Verification items for the finished model (mm, model axes). A direction names the side the tool comes from. Coordinates: 2 decimals unless noted, no trailing zeros. Use CSV: the item, a comma, the result in double quotes. Start each with the question number.
1) Tool access check on faces 1 (the flat face through (-256, -6.969, -14)), 2 (the flat face through (17, 4.65, -13)), 3 (the flat face through (-122.2, 29, -14)), 4 (the flat face through (9, -0.35, -13)), 5 (the flat face through (-256.9, -4.719, -11.7)). Record the directions out of +Z, -Z, +X, -X, +Y, -Y that give a thin tool (end or side, any length) a straight path to the whole face; none if there is none.
2) Go/stop test with flat-tipped pins: pin 1 (4.5 mm diameter, centred on y = 12.5, z = -11, fed in from +X); pin 2 (8 mm diameter, centred on x = -131.5, z = -16.5, fed in from +Y); pin 3 (3.5 mm diameter, centred on x = 13.66, z = -13.5, fed in from -Y). Record where each tip stops, or that it passes through.
3) Scan lines: line 1 along X through (y, z) = (29.5, -16); line 2 along Y through (x, z) = (-69.2, -17.5); line 3 along Y through (x, z) = (-67, -7.5). Record each from-to range of solid material in increasing order.
4) Release check for a two-part mould opening along X. For faces 6 (the flat face through (-259.656, -7, -13)), 7 (the flat face through (18.69, 2, -13)), 8 (the flat face through (-200.81, 14, -14)) record: released by +X, released by -X, zero draft, split by the parting line, or undercut.
from build123d import *

# Parameters (mm, degrees)
BOSS_EXTRUDE14_DEPTH            = 15
SKETCH9_W                       = 10.305582395
SKETCH9_H                       = 5
BOSS_EXTRUDE15_DEPTH            = 15
BOSS_EXTRUDE16_START            = -15
BOSS_EXTRUDE16_OUTLINE_R        = 4
BOSS_EXTRUDE16_DEPTH            = 15
FILLET1_R                       = 4
CUT_EXTRUDE2_DEPTH              = 2.25
CUT_EXTRUDE3_DEPTH              = 2.25
F_3_0MM_DOWEL_HOLE1_D           = 3
F_3_0MM_DOWEL_HOLE1_CSINK_D     = 3.05
F_3_0MM_DOWEL_HOLE1_CSINK_ANGLE = 90
SKETCH16_R                      = 1.5
CUT_EXTRUDE4_DEPTH              = 265.853431953


# Read off the part's stored shape, not the designer's step: Boss-Extrude14, Boss-Extrude16
with BuildPart() as part:
    # Boss-Extrude14 outline → Boss-Extrude14 (new body)
    with BuildSketch(Plane(origin=(0, 0, -6), x_dir=(-1, 0, 0), z_dir=(0, 0, -1))):
        with BuildLine():
            Line((249.35, -9.718799499), (249.35, 0.281200501))
            Line((249.35, 0.281200501), (236.35, 2.868680647))
            add(Edge.make_bspline(
                [(113.156309789, 25.751987472), (114.460208978, 25.59959164), (120.100287856, 24.908577179), (128.609098159, 23.664110071), (140.134091586, 21.688830409), (153.008895552, 19.221496185), (168.538046321, 16.015172699), (182.477939999, 13.172125281), (193.559005245, 11.111240975), (201.981640704, 9.637661129), (210.486612866, 8.154956205), (219.063637957, 6.591746422), (227.68151116, 4.874943897), (233.474971, 3.568357951), (236.35, 2.868680647)],
                knots=[0.109458463, 0.109458463, 0.109458463, 0.109458463, 0.130371933, 0.200030506, 0.247022058, 0.318338141, 0.412321245, 0.506304349, 0.553295901, 0.600287453, 0.647279005, 0.694270557, 0.741262109, 0.788253661, 0.788253661, 0.788253661, 0.788253661], degree=3))
            add(Edge.make_bspline(
                [(76.45, 28.125418087), (94.882372903, 27.862574162), (113.156309789, 25.751987472)],
                knots=[0, 0, 0, 0.632722323, 0.632722323, 0.632722323], degree=2))
            add(Edge.make_bspline(
                [(66.284340587, 28.219952736), (67.129544996, 28.219602739), (68.818588071, 28.215923169), (71.36030606, 28.198672488), (73.903160315, 28.169538769), (75.601337427, 28.141603711), (76.45, 28.125418087)],
                knots=[0.875312122, 0.875312122, 0.875312122, 0.875312122, 0.888961276, 0.902610431, 0.916259586, 0.92990874, 0.92990874, 0.92990874, 0.92990874], degree=3))
            add(Edge.make_bspline(
                [(-4.147448422, 10.754973325), (-3.746592061, 11.135583203), (-2.910664688, 11.873123525), (-1.8664669, 12.676265805), (-1.020623492, 13.271741618), (-0.136993775, 13.859475937), (1.465019188, 14.831768722), (3.815921844, 16.045559455), (7.753628889, 17.758192835), (13.256195767, 19.698691993), (21.152959065, 21.952811545), (30.479838242, 24.122904012), (39.4239247, 25.749420494), (47.205771024, 26.831006606), (53.324700432, 27.499051298), (58.631201034, 27.906826379), (62.977570557, 28.125868706), (65.18464413, 28.194929818), (66.284340587, 28.219952736)],
                knots=[0.135157363, 0.135157363, 0.135157363, 0.135157363, 0.162214964, 0.189272566, 0.201061372, 0.214590172, 0.243387768, 0.297502971, 0.351618174, 0.459848579, 0.568078984, 0.676309389, 0.784539795, 0.838654997, 0.8927702, 0.946885402, 0.973943004, 1.001000605, 1.001000605, 1.001000605, 1.001000605], degree=3))
            add(Edge.make_bspline(
                [(-8.702959439, 4.575291566), (-6.890883257, 8.114910032), (-4.147448422, 10.754973325)],
                knots=[0, 0, 0, 0.636944249, 0.636944249, 0.636944249], degree=2))
            add(Edge.make_bspline(
                [(-8.702959439, 4.575291566), (-8.771267052, 4.454592439), (-8.899970783, 4.219174636), (-9.174274638, 3.674724808), (-9.523622742, 2.874059155), (-9.910621046, 1.66916954), (-10.123727188, 0.514933148), (-10.179306724, -0.189247064), (-10.188216911, -0.35)],
                knots=[0, 0, 0, 0, 0.000508489, 0.001016978, 0.002033955, 0.003050933, 0.00394155, 0.004195794, 0.004195794, 0.004195794, 0.004195794], degree=3))
            Line((-10.188216911, -0.35), (0, -0.35))
            add(Edge.make_bspline(
                [(0, -0.35), (3.178862469, 6.495343287), (8.987756305, 8.032168144), (22.140633739, 13.071207305), (43.250433247, 17.69324185), (66.39602757, 18.219905629)],
                knots=[0, 0, 0, 0, 0, 0, 1, 1, 1, 1, 1, 1], degree=5))
            add(Edge.make_bspline(
                [(66.39602757, 18.219905629), (73.079858249, 18.217137873), (79.768873399, 18.101745103), (86.45, 17.815976098)],
                knots=[0.875945967, 0.875945967, 0.875945967, 0.875945967, 0.985673704, 0.985673704, 0.985673704, 0.985673704], degree=3))
            Line((86.45, 17.815976098), (89.45, 17.675984992))
            ThreePointArc((89.45, 17.675984992), (90.756210616, 17.607556707), (92.062168571, 17.534464817))
            add(Edge.make_bspline(
                [(92.062168571, 17.534464817), (95.665977641, 17.334138157), (108.464938821, 16.428798519), (140.620964858, 12.117510077), (187.478425037, 1.167330167), (226.131267819, -4.204534739), (244.655582392, -9.718799508)],
                knots=[0, 0, 0, 0, 0.05922822, 0.210539222, 0.531730365, 0.848733007, 0.848733007, 0.848733007, 0.848733007], degree=3))
            Line((244.655582392, -9.718799508), (249.35, -9.718799499))
        make_face()
    extrude(amount=BOSS_EXTRUDE14_DEPTH)

    # Sketch9 → Boss-Extrude15 (add)
    with BuildSketch(Plane.XY.offset(-6)):
        with BuildLine():
            add(Edge.make_bspline(
                [(8.702959439, 4.575291566), (8.771267052, 4.454592439), (8.899970783, 4.219174636), (9.174274638, 3.674724808), (9.523622742, 2.874059155), (9.910621046, 1.66916954), (10.123727188, 0.514933148), (10.179306724, -0.189247064), (10.188216911, -0.35)],
                knots=[0, 0, 0, 0, 0.000508489, 0.001016978, 0.002033955, 0.003050933, 0.00394155, 0.004195794, 0.004195794, 0.004195794, 0.004195794], degree=3))
            Line((10.188216911, -0.35), (18.69, -0.35))
            Line((18.69, -0.35), (18.69, 4.65))
            Line((18.69, 4.65), (8.664557691, 4.65))
            add(Edge.make_bspline(
                [(8.702959439, 4.575291566), (8.683810567, 4.612696009), (8.664557691, 4.65)],
                knots=[0, 0, 0, 0.006730823, 0.006730823, 0.006730823], degree=2))
        make_face()
        with Locations((-254.502791198, -7.218799499)):
            Rectangle(SKETCH9_W, SKETCH9_H)
    extrude(amount=-BOSS_EXTRUDE15_DEPTH)

    # Boss-Extrude16 outline → Boss-Extrude16 (add)
    # profile 1 of 3: a face of its own
    with BuildSketch(Plane.XY.offset(-6).offset(BOSS_EXTRUDE16_START)):
        with BuildLine():
            add(Edge.make_bspline(
                [(-200.81, 9.843246703), (-201.204842604, 9.774216263), (-204.419312994, 9.212692224), (-210.400725126, 8.169929349), (-216.031409877, 7.144376286), (-218.81, 6.615762453)],
                knots=[0.593701678, 0.593701678, 0.593701678, 0.593701678, 0.600287453, 0.647279005, 0.69284692, 0.69284692, 0.69284692, 0.69284692], degree=3))
            Line((-200.81, 9.843246703), (-200.81, 22.86245595))
            Line((-200.81, 22.86245595), (-218.81, 22.86245595))
            Line((-218.81, 22.86245595), (-218.81, 6.615762453))
        make_face()
        with Locations((-209.81, 15.36245595)):
            Circle(BOSS_EXTRUDE16_OUTLINE_R, mode=Mode.SUBTRACT)
    # profile 2 of 3: a face of its own
    with BuildSketch(Plane.XY.offset(-6).offset(BOSS_EXTRUDE16_START)):
        with BuildLine():
            add(Edge.make_bspline(
                [(-122.199999995, 24.58006078), (-124.804407306, 24.210507661), (-130.301243555, 23.374091651), (-136.28735582, 22.348126136), (-139.677142176, 21.735093133), (-140.2, 21.639813309)],
                knots=[0.15796988, 0.15796988, 0.15796988, 0.15796988, 0.200030506, 0.247022058, 0.255600029, 0.255600029, 0.255600029, 0.255600029], degree=3))
            Line((-122.199999995, 24.58006078), (-122.2, 37.420573855))
            Line((-122.2, 37.420573855), (-140.2, 37.420573855))
            Line((-140.2, 37.420573855), (-140.2, 21.639813309))
        make_face()
        with Locations((-131.2, 29.920573855)):
            Circle(BOSS_EXTRUDE16_OUTLINE_R, mode=Mode.SUBTRACT)
    # profile 3 of 3: a face of its own
    with BuildSketch(Plane.XY.offset(-6).offset(BOSS_EXTRUDE16_START)):
        with BuildLine():
            Line((-60.199999997, 27.980034372), (-60.2, 43.08620947))
            Line((-60.2, 43.08620947), (-78.2, 43.08620947))
            Line((-78.2, 43.08620947), (-78.199999995, 28.096292606))
            add(Edge.make_bspline(
                [(-76.45, 28.125418087), (-77.325178587, 28.112938121), (-78.199999995, 28.096292606)],
                knots=[0, 0, 0, 0.030041983, 0.030041983, 0.030041983], degree=2))
            add(Edge.make_bspline(
                [(-66.284340587, 28.219952736), (-67.129544996, 28.219602739), (-68.818588071, 28.215923169), (-71.36030606, 28.198672488), (-73.903160315, 28.169538769), (-75.601337427, 28.141603711), (-76.45, 28.125418087)],
                knots=[0.875312122, 0.875312122, 0.875312122, 0.875312122, 0.888961276, 0.902610431, 0.916259586, 0.92990874, 0.92990874, 0.92990874, 0.92990874], degree=3))
            add(Edge.make_bspline(
                [(-60.199999997, 27.980034372), (-61.122523668, 28.03215495), (-63.139027933, 28.130920838), (-65.18464413, 28.194929818), (-66.284340587, 28.219952736)],
                knots=[0.950844173, 0.950844173, 0.950844173, 0.950844173, 0.973943004, 1.001000605, 1.001000605, 1.001000605, 1.001000605], degree=3))
        make_face()
        with Locations((-69.2, 35.58620947)):
            Circle(BOSS_EXTRUDE16_OUTLINE_R, mode=Mode.SUBTRACT)
    extrude(amount=BOSS_EXTRUDE16_DEPTH)

    # Fillet1
    fillet1_edges = [part.edges().sort_by_distance(p)[0] for p in [
        (-200.81, 22.86245595, -13.5),
        (-218.81, 22.86245595, -13.5),
        (-140.2, 37.420573855, -13.5),
        (-122.2, 37.420573855, -13.5),
        (-60.2, 43.08620947, -13.5),
        (-78.2, 43.08620947, -13.5),
    ]]
    fillet(fillet1_edges, radius=FILLET1_R)

    # Sketch12 → Cut-Extrude2 (cut)
    with BuildSketch(Plane(origin=(0, -4.718799499, 0), x_dir=(1, 0, 0), z_dir=(0, 1, 0))):
        with BuildLine():
            Line((-252.85, 13.5), (-251, 13.5))
            Line((-251, 13.5), (-252.672949017, 16.4))
            Line((-252.672949017, 16.4), (-256.027050983, 16.4))
            Line((-256.027050983, 16.4), (-257.7, 13.5))
            Line((-257.7, 13.5), (-255.85, 13.5))
            ThreePointArc((-255.85, 13.5), (-254.35, 15), (-252.85, 13.5))
        make_face()
        with BuildLine():
            Line((-252.672949017, 10.6), (-251, 13.5))
            Line((-251, 13.5), (-252.85, 13.5))
            ThreePointArc((-252.85, 13.5), (-254.35, 12), (-255.85, 13.5))
            Line((-255.85, 13.5), (-257.7, 13.5))
            Line((-257.7, 13.5), (-256.027050983, 10.6))
            Line((-256.027050983, 10.6), (-252.672949017, 10.6))
        make_face()
        with BuildLine():
            ThreePointArc((-255.85, 13.5), (-254.35, 12), (-252.85, 13.5))
            Line((-252.85, 13.5), (-254.35, 13.5))
            Line((-254.35, 13.5), (-255.85, 13.5))
        make_face()
    extrude(amount=-CUT_EXTRUDE2_DEPTH, mode=Mode.SUBTRACT)

    # Sketch14 → Cut-Extrude3 (cut)
    with BuildSketch(Plane(origin=(0, 4.65, 0), x_dir=(1, 0, 0), z_dir=(0, 1, 0))):
        with BuildLine():
            ThreePointArc((13.664557695, 15), (14.725217866, 14.560660172), (15.164557695, 13.5))
            Line((15.164557695, 13.5), (17.014557695, 13.5))
            Line((17.014557695, 13.5), (15.341608678, 16.4))
            Line((15.341608678, 16.4), (13.664557695, 16.4))
            Line((13.664557695, 16.4), (13.664557695, 15))
        make_face()
        with BuildLine():
            Line((10.314557695, 13.5), (12.164557695, 13.5))
            ThreePointArc((12.164557695, 13.5), (12.603897523, 14.560660172), (13.664557695, 15))
            Line((13.664557695, 15), (13.664557695, 16.4))
            Line((13.664557695, 16.4), (11.987506712, 16.4))
            Line((11.987506712, 16.4), (10.314557695, 13.5))
        make_face()
        with BuildLine():
            Line((11.987506712, 10.6), (13.664557695, 10.6))
            Line((13.664557695, 10.6), (13.664557695, 12))
            ThreePointArc((13.664557695, 12), (12.603897523, 12.439339828), (12.164557695, 13.5))
            Line((12.164557695, 13.5), (10.314557695, 13.5))
            Line((10.314557695, 13.5), (11.987506712, 10.6))
        make_face()
        with BuildLine():
            Line((13.664557695, 12), (13.664557695, 10.6))
            Line((13.664557695, 10.6), (15.341608678, 10.6))
            Line((15.341608678, 10.6), (17.014557695, 13.5))
            Line((17.014557695, 13.5), (15.164557695, 13.5))
            ThreePointArc((15.164557695, 13.5), (14.725217866, 12.439339828), (13.664557695, 12))
        make_face()
    extrude(amount=-CUT_EXTRUDE3_DEPTH, mode=Mode.SUBTRACT)

    # Ø3.0mm Dowel Hole1 (through all)
    with Locations(Plane(origin=(0, 4.65, 0), x_dir=(1, 0, 0), z_dir=(0, 1, 0))):
        with Locations((13.664557695, 13.5)):
            CounterSinkHole(F_3_0MM_DOWEL_HOLE1_D / 2, F_3_0MM_DOWEL_HOLE1_CSINK_D / 2, counter_sink_angle=F_3_0MM_DOWEL_HOLE1_CSINK_ANGLE)

    # Sketch16 → Cut-Extrude4 (cut, through all)
    with BuildSketch(Plane(origin=(0, -4.718799499, 0), x_dir=(1, 0, 0), z_dir=(0, 1, 0))):
        with Locations(Location((-254.35, 13.5, 0), (0, 0, 180))):
            Circle(SKETCH16_R)
    extrude(amount=-CUT_EXTRUDE4_DEPTH, mode=Mode.SUBTRACT)


solid = part.part
Answers follow:
1,face 1,"+Y"
1,face 2,"+Z, -Z, +X, +Y"
1,face 3,"+Z, -Z, +Y"
1,face 4,"+Z, -Z, +X, -Y"
1,face 5,"+Z, -Z, -X, +Y"
2,pin 1,"stops at x = 4.66"
2,pin 2,"stops at y = 37.42"
2,pin 3,"stops at y = -0.35"
3,line 1,"x = -140.2 to -135.18, -127.22 to -122.2, -78.2 to -60.2"
3,line 2,"y = 18.21 to 31.59, 39.59 to 43.09"
3,line 3,"y = 18.22 to 32.25, 38.93 to 43.09"
4,face 6,"released by -X"
4,face 7,"released by +X"
4,face 8,"undercut"
